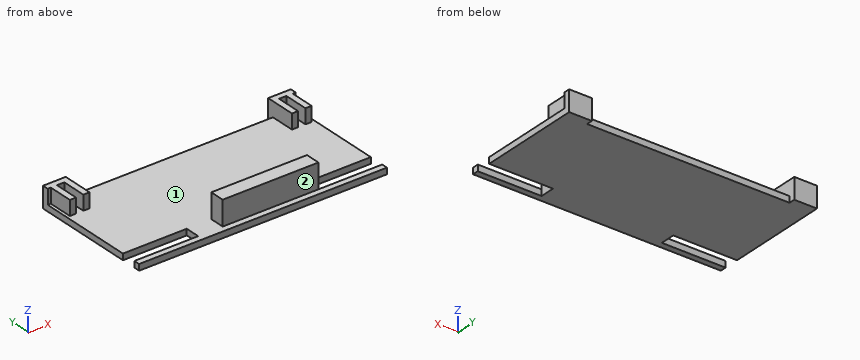
```python
from build123d import *

# Parameters (mm, degrees)
SKETCH1_W           = 50.5
SKETCH1_H           = 24
BOSS_EXTRUDE1_DEPTH = 1.25
SKETCH2_W           = 1.25
SKETCH2_H           = 3
BOSS_EXTRUDE2_DEPTH = 5
SKETCH3_W           = 13
SKETCH3_H           = 3
CUT_EXTRUDE1_DEPTH  = 1.25
SKETCH5_W           = 4.628536498
SKETCH5_H           = 4.25
BOSS_EXTRUDE3_DEPTH = 1.25
SKETCH9_W           = 19.5
SKETCH9_H           = 3
BOSS_EXTRUDE5_DEPTH = 5


with BuildPart() as part:
    # Sketch1 → Boss-Extrude1 (new body)
    with BuildSketch(Plane.XY):
        with Locations((24, 12)):
            Rectangle(SKETCH1_W, SKETCH1_H)
    extrude(amount=BOSS_EXTRUDE1_DEPTH)

    # Sketch2 → Boss-Extrude2 (add)
    with BuildSketch(Plane(origin=(0, 24, 0), x_dir=(1, 0, 0), z_dir=(0, 1, 0))):
        with Locations((47.996463502, -2.75)):
            Rectangle(SKETCH2_W, SKETCH2_H)
        with Locations((45.246463502, -2.75)):
            Rectangle(SKETCH2_W, SKETCH2_H)
        with Locations((2.753536498, -2.75)):
            Rectangle(SKETCH2_W, SKETCH2_H)
        with Locations((0.003536498, -2.75)):
            Rectangle(SKETCH2_W, SKETCH2_H)
    extrude(amount=-BOSS_EXTRUDE2_DEPTH)

    # Sketch3 → Cut-Extrude1 (cut)
    with BuildSketch(Plane(origin=(0, 0, 0), x_dir=(-1, 0, 0), z_dir=(0, 0, -1))):
        with Locations((-42.75, 2.75)):
            Rectangle(SKETCH3_W, SKETCH3_H)
        with Locations((-5.25, 2.75)):
            Rectangle(SKETCH3_W, SKETCH3_H)
    extrude(amount=-CUT_EXTRUDE1_DEPTH, mode=Mode.SUBTRACT)

    # Sketch5 → Boss-Extrude3 (add)
    with BuildSketch(Plane(origin=(0, 24, 0), x_dir=(1, 0, 0), z_dir=(0, 1, 0))):
        with Locations((1.064268249, -2.125)):
            Rectangle(SKETCH5_W, SKETCH5_H)
        with Locations((46.935731751, -2.125)):
            Rectangle(SKETCH5_W, SKETCH5_H)
    extrude(amount=BOSS_EXTRUDE3_DEPTH)

    # Sketch9 → Boss-Extrude5 (add)
    with BuildSketch(Plane.XY.offset(1.25)):
        with Locations((26.5, 2.75)):
            Rectangle(SKETCH9_W, SKETCH9_H)
    extrude(amount=BOSS_EXTRUDE5_DEPTH)


solid = part.part
```
The listing builds one solid part. Answer for the finished solid, in the listing's coordinates (mm). Face numbers are marked on the shaded views. Coordinates: 2 decimals unless noted, no trailing zeros. Write each loop counter-clockwise with the first axis right and the second up, starting at its lowest first coordinate (ties: lowest second). Pieces come first, ordered by that corner, then holes.
Q1. The mould has two halves that part along X. Classify the marked faces 1 and 2: released by +X, released by -X, zero draft, split by the parting line, or undercut.
Returned:
face 1: undercut
face 2: zero draft
Q2. Find the intervals of material crossed by line 1 along Z through (x, y) = (16, 4.5); line 2 along Y through (x, z) = (45, 3.5); line 3 along X through (y, z) = (3.75, 1), in increasing order.
Returned:
line 1: z = 0 to 1.25
line 2: y = 19 to 25.25
line 3: x = 11.75 to 36.25
Q3. Section B-B, the plane x = 4 is taken. Write down the section's boundary in (y, z).
Returned:
outline: (0, 0) - (1.25, 0) - (1.25, 1.25) - (0, 1.25) - close; (4.25, 0) - (24, 0) - (24, 1.25) - (4.25, 1.25) - close
Q4. Section A-A, the plane z = 3.75 is taken. Write down the section's boundary in (x, y), then the cut area to 3 significant figures.
Returned:
outline: (-1.25, 24) - (-0.62, 24) - (-0.62, 19) - (0.63, 19) - (0.63, 24) - (2.13, 24) - (2.13, 19) - (3.38, 19) - (3.38, 25.25) - (-1.25, 25.25) - close; (16.75, 1.25) - (36.25, 1.25) - (36.25, 4.25) - (16.75, 4.25) - close; (44.62, 19) - (45.87, 19) - (45.87, 24) - (47.37, 24) - (47.37, 19) - (48.62, 19) - (48.62, 24) - (49.25, 24) - (49.25, 25.25) - (44.62, 25.25) - close
area: 95.1 mm2
Q5. Section C-C, the plane y = 21.75 is taken. Write down the section's boundary in (x, z), then the cut area to 3 significant figures.
Returned:
outline: (-1.25, 0) - (49.25, 0) - (49.25, 1.25) - (48.62, 1.25) - (48.62, 4.25) - (47.37, 4.25) - (47.37, 1.25) - (45.87, 1.25) - (45.87, 4.25) - (44.62, 4.25) - (44.62, 1.25) - (3.38, 1.25) - (3.38, 4.25) - (2.13, 4.25) - (2.13, 1.25) - (0.63, 1.25) - (0.63, 4.25) - (-0.62, 4.25) - (-0.62, 1.25) - (-1.25, 1.25) - close
area: 78.1 mm2
Q6. Section D-D, the plane x = 18 is taken. Write down the section's boundary in (y, z), then the cut area to 3 significant figures.
Returned:
outline: (0, 0) - (24, 0) - (24, 1.25) - (4.25, 1.25) - (4.25, 6.25) - (1.25, 6.25) - (1.25, 1.25) - (0, 1.25) - close
area: 45.0 mm2
Q7. Given P1, Ø3, axis at x = 9.5, z = 1.5, coming from the -Y side; P2, Ø1.4, axis at x = 46.5, y = 21.5, coming from the +Z side; P3, Ø3.5, axis at y = 3, z = 4.5, coming from the -X side; P4, Ø2.5, axis at y = 3, z = 3, coming from the +X side, each flat-ended and moving along its own axis, determine where each tip first touches the part or whether it passes through.
Returned:
P1: stops at y = 0
P2: stops at z = 4.25
P3: stops at x = 16.75
P4: stops at x = 36.25
